Autodesk Inventor part; units mm, degrees
ref_plane "YZ Plane" through (0, 0, 0) normal (1, 0, 0) x (0, 1, 0)
ref_plane "XZ Plane" through (0, 0, 0) normal (0, 1, 0) x (-1, 0, 0)
ref_plane "XY Plane" through (0, 0, 0) normal (0, 0, 1) x (1, 0, 0)
sketch "Boceto1" plane through (0, 0, 0) normal (0, 1, 0) x (-1, 0, 0)
  circle A0 centre (0, 0) radius 5
  dimension "d0" = 10
extrude "Extrusión1" add sketch "Boceto1" along normal blind 4
sketch "Boceto2" plane through (0, 4, 0) normal (0, 1, 0) x (1, 0, 0)
  circle A0 centre (0, 0) radius 0.65
  dimension "d3" = 1.3
extrude "Extrusión2" add sketch "Boceto2" along normal blind 9
sketch "Boceto3" plane through (0, 13, 0) normal (0, 1, 0) x (1, 0, 0)
  circle A0 centre (0, 0) radius 0.65
  line L0 (0, -0.65) -> (0, 0.65)
  circle A1 centre (0, 0) radius 0.65
extrude "Extrusión3" cut sketch "Boceto3" against normal blind 1.5 contours L0 A0 picked at (-0.0519, -0.2104)
properties part number "ServoPot"
Check sheet for the modelled part. Datum: model origin and axes. Units: mm. A direction names the side the tool comes from. Coordinates: 2 decimals unless noted, no trailing zeros. Loops run counter-clockwise (first coordinate to the right, second up) from the corner with the lowest first, then second, coordinate; pieces in that order, holes last.
1) Access from +Z, -Z, +X, -X, +Y, -Y to the whole of each face (thin tool, end or side, straight path). Record for faces 1 (the face through (0, 12, 0)), 2 (the face through (1.08, 1.97, 4.88)), 3 (the face through (0.62, 8.44, 0.2)).
2) Material ranges on probe 1 along Y at (x, z) = (2.5, 3); probe 2 along X at (y, z) = (3, -0.25); probe 3 along Z at (x, y) = (1.5, 2.5), recorded low to high.
3) Sectioned sample at A-A (z = 0). Record the boundary of the cut face in (x, y).
4) Sectioned sample at D-D (y = 1.75). Record the boundary of the cut face in (x, z), and give its area (3 significant figures).
5) Gauge pin test, flat ends, axial feed: pin 1 (3 mm diameter, centred on x = -2, y = 4.5, fed in from -Z); pin 2 (5 mm diameter, centred on x = 1.5, z = -2, fed in from +Y); pin 3 (6 mm diameter, centred on x = -1, y = 11, fed in from +Z); pin 4 (1.4 mm diameter, centred on y = 12, z = -0.5, fed in from -X). Record the tip position at first contact, or that the pin passes through.
6) Sectioned sample at C-C (x = -1.75). Record the boundary of the cut face in (y, z), and give its area (3 significant figures).
7) Sectioned sample at B-B (y = 10). Record the boundary of the cut face in (x, z).
Check sheet entries:
1. face 1: +Z, -Z, -X, +Y
1. face 2: +Y, -Y
1. face 3: +Y
2. probe 1: y = 0 to 4
2. probe 2: x = -4.99 to 4.99
2. probe 3: z = -4.77 to 4.77
3. outline: (-5, 0) - (5, 0) - (5, 4) - (0.65, 4) - (0.65, 13) - (0, 13) - (0, 11.5) - (-0.65, 11.5) - (-0.65, 4) - (-5, 4) - close
4. outline: circle Ø10 at (0, 0)
4. area: 78.5 mm2
5. pin 1: stops at z = -4.97
5. pin 2: stops at y = 13
5. pin 3: stops at z = 0.65
5. pin 4: stops at x = -0.65
6. outline: (0, -4.68) - (4, -4.68) - (4, 4.68) - (0, 4.68) - close
6. area: 37.5 mm2
7. outline: circle Ø1.3 at (0, 0)
